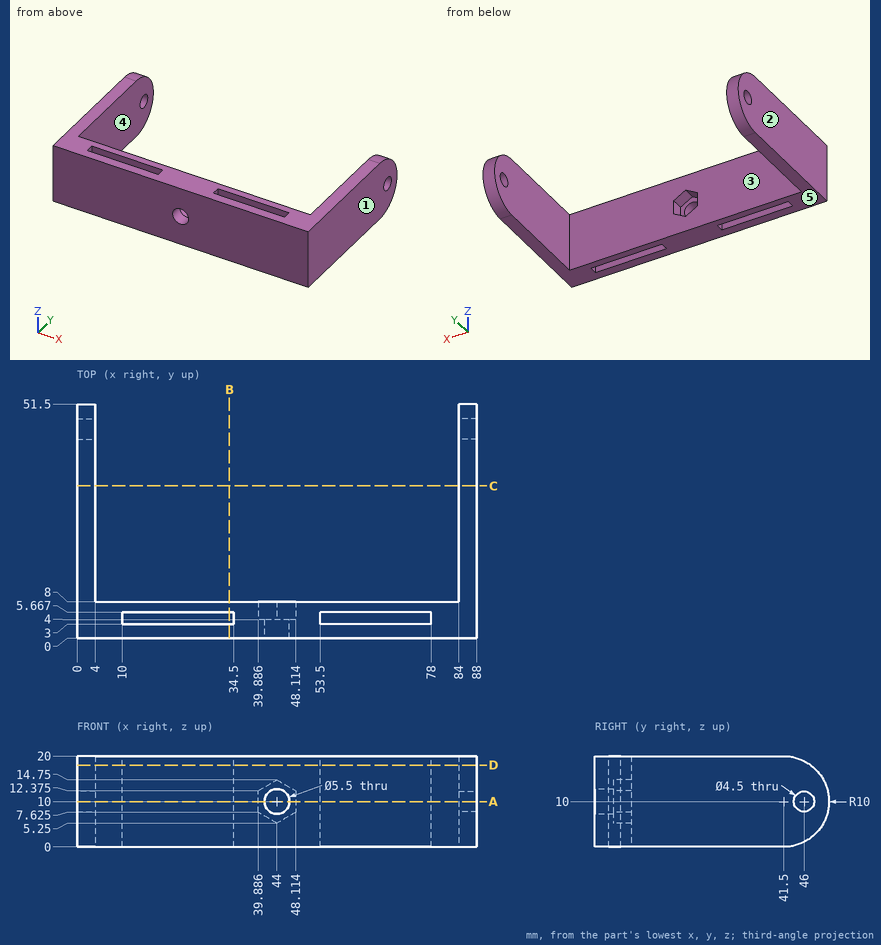
Part print with two shaded views. Sizes in mm from the minimum x, y, z corner. A direction names the side the tool comes from. Coordinates: 2 decimals unless noted, no trailing zeros. Order: outer loops, then holes, each group sorted by start corner. A loop starts at its lowest first (then second) coordinate and runs counter-clockwise, first axis right, second up. Notation, with made-up numbers: M 5,37 L 23,37 A26 ccw 23,75 Z; hole C 20.5,36 d2. An arc over 180 degrees is marked long. Use a Markdown table: item, result.
(1) Flat gauge pin, fed straight in: pin 1 (6.5 mm diameter, centred on x = 44, z = 11.5, fed in from +Y). Where does the tip first touch, or does it go through?
A:
| item | result |
|---|---|
| pin 1 | stops at y = 8 |
(2) Cut at D-D on z = 18. Write the cut outline in (x, y).
A:
| item | result |
|---|---|
| outline | M 0,0 L 88,0 L 88,47.5 L 84,47.5 L 84,8 L 4,8 L 4,47.5 L 0,47.5 Z; hole M 10,3 L 34.5,3 L 34.5,5.67 L 10,5.67 Z; hole M 53.5,3 L 78,3 L 78,5.67 L 53.5,5.67 Z |
(3) Cut at A-A on z = 10. State how many separate pieces and enclosed holes the cut face has.
A:
| item | result |
|---|---|
| separate pieces | 4 |
| enclosed holes | 2 |
(4) Probe L1, parallel to Y at x = 17, z = 3.5; L2, parallel to X at y = 48.5, z = 13; L3, parallel to Z at x = 44, y = 2.55. List the from-to ranges inside material, lowest first.
A:
| item | result |
|---|---|
| L1 | y = 0 to 3, 5.67 to 8 |
| L2 | x = 0 to 4, 84 to 88 |
| L3 | z = 0 to 7.25, 12.75 to 20 |
(5) Pull direction X, two halves, no side cores. Call the marked faces 1, 2 and 3: released by +X, released by -X, zero draft, split by the parting line, or undercut.
A:
| item | result |
|---|---|
| face 1 | released by +X |
| face 2 | released by -X |
| face 3 | undercut |
(6) Cut at B-B on x = 33.5. Write the cut outline in (y, z).
A:
| item | result |
|---|---|
| outline | M 0,0 L 3,0 L 3,20 L 0,20 Z; M 5.67,0 L 8,0 L 8,20 L 5.67,20 Z |
(7) Cut at C-C on y = 33.5. Write the cut outline in (x, z).
A:
| item | result |
|---|---|
| outline | M 0,0 L 4,0 L 4,20 L 0,20 Z; M 84,0 L 88,0 L 88,20 L 84,20 Z |
(8) Tool access for the marked faces 4 and 5: list every direction of +Z, -Z, +X, -X, +Y, -Y with a clear straight run to the whole face (end or side of a thin tool).
A:
| item | result |
|---|---|
| face 4 | +Z, -Z, +Y |
| face 5 | -Z, +X, -X, +Y, -Y |
